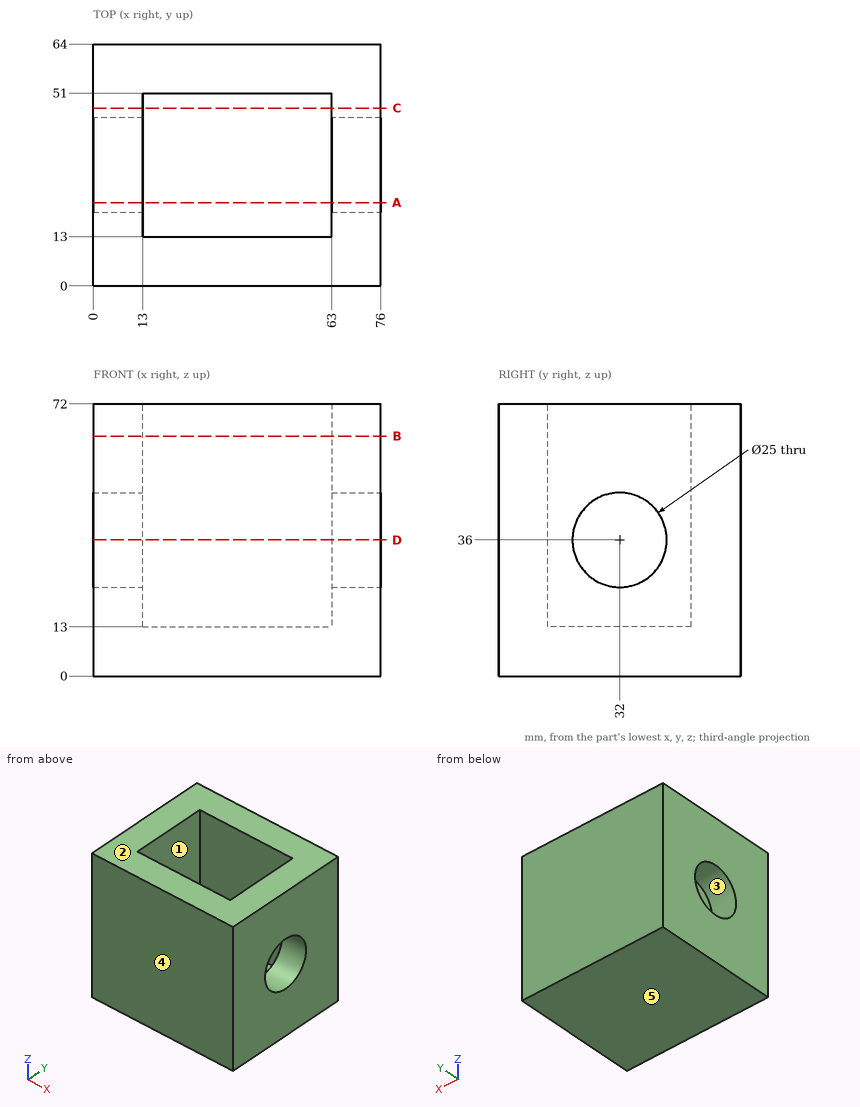
The figure shows three views and two pictorial views of one solid part (mm, origin at its lowest corner). Answer the questions. A direction names the side the tool comes from. Give positions to 0.01 mm unless a question says otherwise; leave off trailing zeros. Loops run counter-clockwise (first coordinate to the right, second up) from the corner with the lowest first, then second, coordinate; pieces in that order, holes last. Notation, with made-up numbers: (-8, -5.75) - (-3, -5.75) arc R27 ccw to (-3, 16.25) - close; hole circle Ø11 at (83.5, 29). An arc over 180 degrees is marked (long way). Answer in a Markdown table with one row per item.
(1) Section C-C (y = 47) is taken. Give the vertices of the cut face in (x, z).
Results list:
| item | result |
|---|---|
| outline | (0, 0) - (76, 0) - (76, 72) - (63, 72) - (63, 13) - (13, 13) - (13, 72) - (0, 72) - close |
(2) For a pull along Y with two mould halves and no side action, classify the marked faces 3, 4 and 5 as pulls with the +Y half, pulls with the -Y half, needs draft (parallel to the pull), parting line crosses it, or undercut.
Results list:
| item | result |
|---|---|
| face 3 | undercut |
| face 4 | pulls with the -Y half |
| face 5 | needs draft |
(3) Consider L1, parallel to Z at x = 7, y = 32; L2, parallel to Y at x = 51.5, z = 59; L3, parallel to Z at x = 17.5, y = 41.5. Determine where each line is inside the solid, lowest interval first. Write a range as [from, to].
Results list:
| item | result |
|---|---|
| L1 | z = [0, 23.5], [48.5, 72] |
| L2 | y = [0, 13], [51, 64] |
| L3 | z = [0, 13] |
(4) Section D-D (z = 36) is taken. Give the vertices of the cut face in (x, y), and give its area (3 significant figures).
Results list:
| item | result |
|---|---|
| outline | (0, 0) - (76, 0) - (76, 19.5) - (63, 19.5) - (63, 13) - (13, 13) - (13, 19.5) - (0, 19.5) - close; (0, 44.5) - (13, 44.5) - (13, 51) - (63, 51) - (63, 44.5) - (76, 44.5) - (76, 64) - (0, 64) - close |
| area | 2,310 mm² |
(5) Section B-B (z = 63.5) is taken. Give the vertices of the cut face in (x, y).
Results list:
| item | result |
|---|---|
| outline | (0, 0) - (76, 0) - (76, 64) - (0, 64) - close; hole (13, 13) - (63, 13) - (63, 51) - (13, 51) - close |
(6) Flat-ended cylindrical pins translate along their axes: pin 1 Ø11.5 at (x, y) = (33, 36.5) entering from +Z; pin 2 Ø22.5 at (y, z) = (32, 36) entering from +X. Find the tip coordinate at first contact, or state that the pin passes through.
Results list:
| item | result |
|---|---|
| pin 1 | stops at z = 13 |
| pin 2 | passes through |
(7) A tool of negligible diameter and unlimited length cuts with its end or side. For the marked faces 1 and 2, from which of +Z, -Z, +X, -X, +Y, -Y can it reach the whole face along a straight path? Write none if from no direction.
Results list:
| item | result |
|---|---|
| face 1 | +Z |
| face 2 | +Z, +X, -X, +Y, -Y |
(8) Section A-A (y = 22) is taken. Give the vertices of the cut face in (x, z), and give its area (3 significant figures).
Results list:
| item | result |
|---|---|
| outline | (0, 0) - (76, 0) - (76, 28.5) - (63, 28.5) - (63, 13) - (13, 13) - (13, 28.5) - (0, 28.5) - close; (0, 43.5) - (13, 43.5) - (13, 72) - (0, 72) - close; (63, 43.5) - (76, 43.5) - (76, 72) - (63, 72) - close |
| area | 2,130 mm² |
